Could you check a few things on this drawing? It's one solid part, dimensions in mm from its lowest x, y, z. Give positions to 0.01 mm unless a question says otherwise; leave off trailing zeros. Loops run counter-clockwise (first coordinate to the right, second up) from the corner with the lowest first, then second, coordinate; pieces in that order, holes last. Notation, with made-up numbers: M 63,78.5 L 79,78.5 A14 cw 79,89.5 Z; hole C -34.75,39.5 d4. An arc over 180 degrees is marked long. Answer as a JSON object with one key per item and string values.
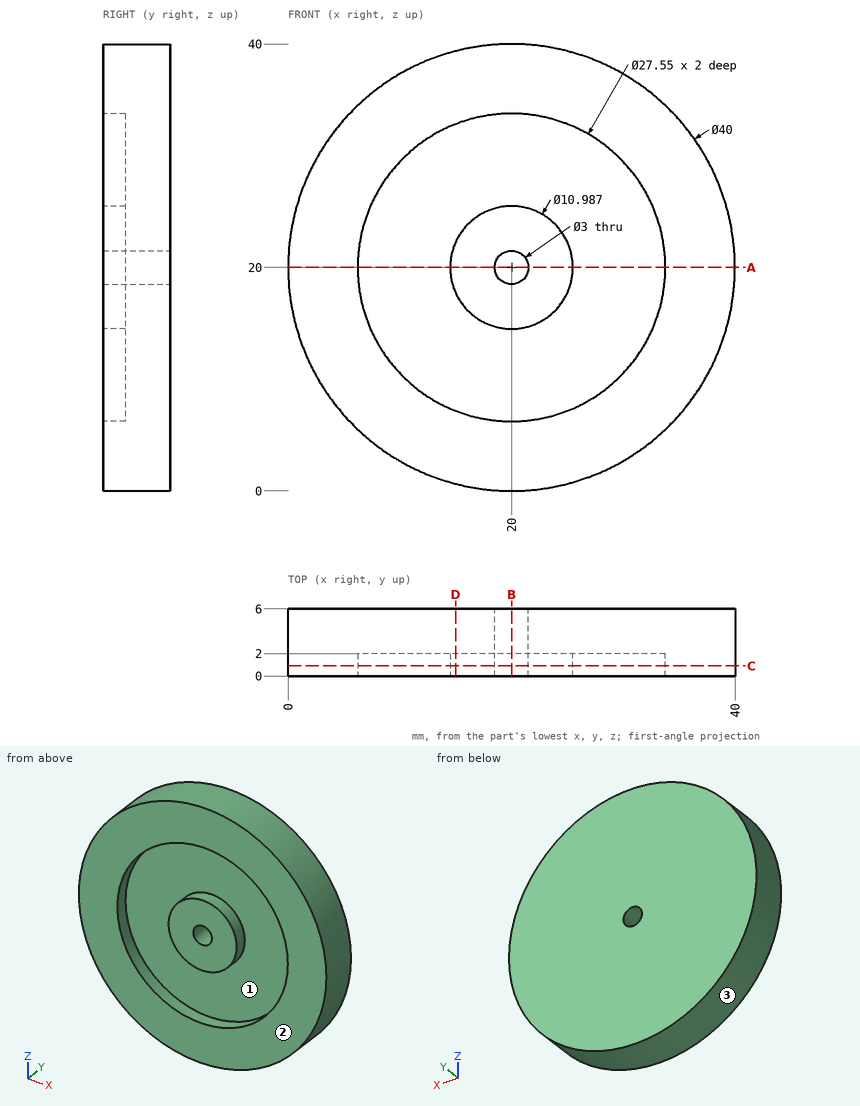
1) Suppose I cut it at D-D, the plane x = 15. Write out the boundary of the cut face in (y, z) (1 decimal), and give its area (3 significant figures).
Answer list:
{"outline": "M 0,0.6 L 6,0.6 L 6,39.4 L 0,39.4 L 0,32.8 L 2,32.8 L 2,22.3 L 0,22.3 L 0,17.7 L 2,17.7 L 2,7.2 L 0,7.2 Z", "area": "190 mm^2"}
2) Please list where these lines run through material, in increasing order: line 1 along Z through (x, y) = (20, 1.65) (1 decimal); line 2 along Z through (x, y) = (20, 2.75); line 3 along Y through (x, z) = (14, 21). Write a range as from..to.
Answer list:
{"line 1": "0..6.2, 14.5..18.5, 21.5..25.5, 33.8..40", "line 2": "0..18.5, 21.5..40", "line 3": "2..6"}
3) Suppose I cut it at A-A, the plane z = 20. Write out the boundary of the cut face in (x, y) (1 decimal), and give its area (3 significant figures).
Answer list:
{"outline": "M 0,0 L 6.2,0 L 6.2,2 L 14.5,2 L 14.5,0 L 18.5,0 L 18.5,6 L 0,6 Z; M 21.5,0 L 25.5,0 L 25.5,2 L 33.8,2 L 33.8,0 L 40,0 L 40,6 L 21.5,6 Z", "area": "189 mm^2"}
4) If we mould it in two halves opening along Z, with no side actions, what happens to the marked faces 1, 2 and 3? For each: +Z half, -Z half, draft (parallel to the pull), parting line (faces both ways), or undercut.
Answer list:
{"face 1": "undercut", "face 2": "draft", "face 3": "parting line"}
5) Will these pins go through, and if not, where does the flat tip stop? pin 1 Ø1 at (y, z) = (4.5, 31) entering from -X; pin 2 Ø3 at (x, y) = (32.5, 3) entering from -Z.
Answer list:
{"pin 1": "x = 2.98", "pin 2": "z = 3.3"}
6) Suppose I cut it at B-B, the plane x = 20. Write out the boundary of the cut face in (y, z) (1 decimal).
Answer list:
{"outline": "M 0,0 L 6,0 L 6,18.5 L 0,18.5 L 0,14.5 L 2,14.5 L 2,6.2 L 0,6.2 Z; M 0,21.5 L 6,21.5 L 6,40 L 0,40 L 0,33.8 L 2,33.8 L 2,25.5 L 0,25.5 Z"}
7) Suppose I cut it at C-C, the plane y = 0.9. Give the number of separate pieces and of enclosed holes in the cut face, and give its area (3 significant figures).
Answer list:
{"separate pieces": "2", "enclosed holes": "2", "area": "748 mm^2"}
